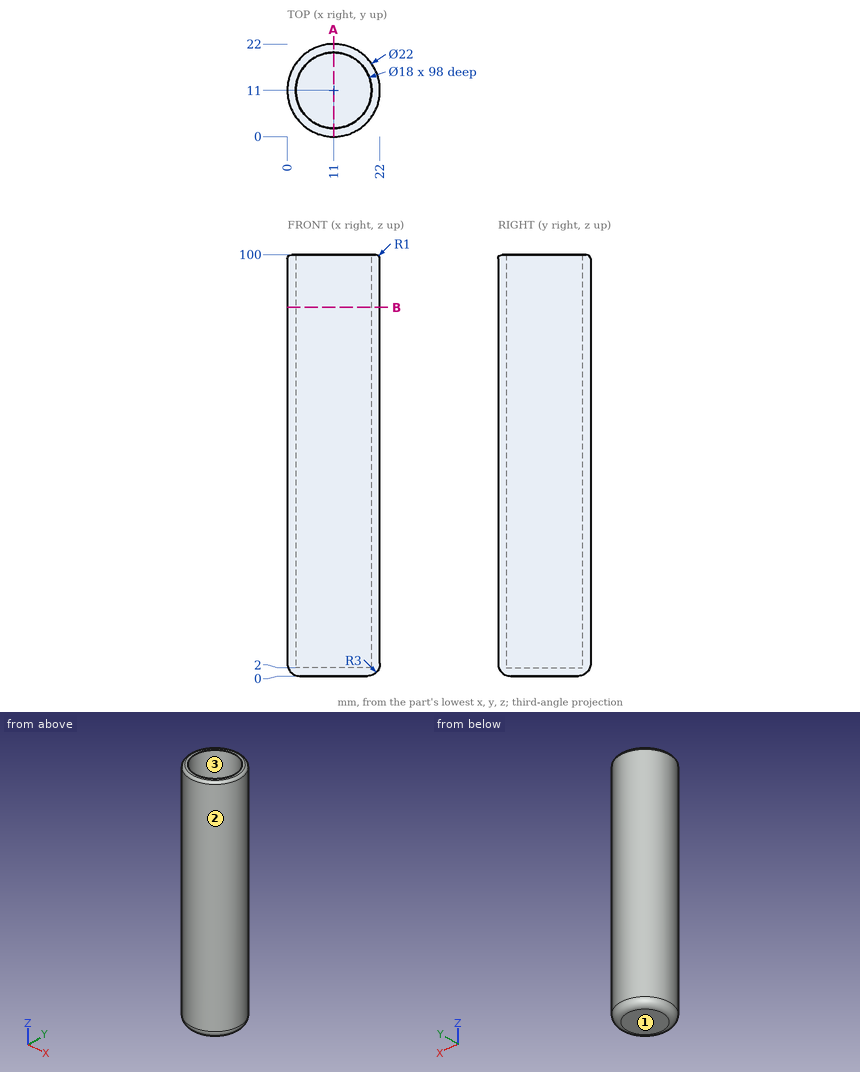
Geometry check sheet. Reference: drawing and pictorial views, mm from the part's lowest x, y, z. Give positions to 0.01 mm unless a question says otherwise; leave off trailing zeros. Order: outer loops, then holes, each group sorted by start corner. A loop starts at its lowest first (then second) coordinate and runs counter-clockwise, first axis right, second up. Notation, with made-up numbers: (62.25, 31) -> (121.25, 31) arc R27 ccw to (121.25, 70) -> close; hole circle Ø11 at (-19.5, 86.25). An arc over 180 degrees is marked (long way). Use CSV: the item, a comma, the result in double quotes. Start each with the question number.
1) Material ranges on line 1 (Y direction, x = 11, z = 77); line 2 (Z direction, x = 13.75, y = 15); line 3 (Y direction, x = 18, z = 44.5), recorded low to high. Write a range as from..to.
2) Go/stop test with flat-tipped pins: P1, Ø3, axis at x = 15, z = 13.5, coming from the +Y side; P2, Ø8, axis at x = 14.5, z = 64.5, coming from the +Y side; P3, Ø1, axis at x = 17, y = 10.5, coming from the +Z side; P4, Ø1, axis at y = 16.5, z = 36, coming from the +X side. Record where each tip stops, or that it passes through.
3) Sectioned sample at A-A, the plane x = 11. Record the boundary of the cut face in (y, z), plus the area to 3 significant figures.
4) Mould release check, pull along Y, two halves, no side actions. Record for the marked faces 1, 2 and 3: released by +Y, released by -Y, zero draft, split by the parting line, or undercut.
5) Sectioned sample at B-B, the plane z = 87.5. Record the boundary of the cut face in (x, y), plus the area to 3 significant figures.
Recorded:
1,line 1,"0..2, 20..22"
1,line 2,"0..2"
1,line 3,"2.51..5.34, 16.66..19.49"
2,P1,"y = 21.71"
2,P2,"y = 22"
2,P3,"z = 2"
2,P4,"x = 20.8"
3,outline,"(0, 3) arc R3 ccw to (3, 0) -> (19, 0) arc R3 ccw to (22, 3) -> (22, 99) arc R1 ccw to (21, 100) -> (20, 100) -> (20, 2) -> (2, 2) -> (2, 100) -> (1, 100) arc R1 ccw to (0, 99) -> close"
3,area,"432 mm2"
4,face 1,"zero draft"
4,face 2,"split by the parting line"
4,face 3,"undercut"
5,outline,"circle Ø22 at (11, 11); hole circle Ø18 at (11, 11)"
5,area,"126 mm2"
